Verification items for the finished model (mm, model axes). A direction names the side the tool comes from. Give positions to 0.01 mm unless a question says otherwise; leave off trailing zeros. Loops run counter-clockwise (first coordinate to the right, second up) from the corner with the lowest first, then second, coordinate; pieces in that order, holes last. Notation, with made-up numbers: M 82.25,-19.75 L 134.25,-19.75 A16 ccw 134.25,-1.75 Z; hole C 89,-36 d9. An arc over 180 degrees is marked long. Answer in a Markdown table with one row per item.
```python
from build123d import *

# Parameters (mm, degrees)
F0_R     = 17.5
F1_DEPTH = 2.5
F2_R     = 3
F3_DEPTH = 5


with BuildPart() as f1:
    # F0 (on Front) → F1 (new body, symmetric)
    with BuildSketch(Plane.XZ):
        Circle(F0_R)
        with BuildLine():
            ThreePointArc((-3.4692543384, -12.0089247785), (-6.25, -10.8253175473), (-8.6654067611, -9.0089247785))
            Line((-8.6654067611, -9.0089247785), (-7.8895788335, -7.6651513899))
            ThreePointArc((-7.8895788335, -7.6651513899), (-9.5262794416, -5.5), (-10.5830052443, -3))
            Line((-10.5830052443, -3), (-12.1346610995, -3))
            ThreePointArc((-12.1346610995, -3), (-12.5, 0), (-12.1346610995, 3))
            Line((-12.1346610995, 3), (-10.5830052443, 3))
            ThreePointArc((-10.5830052443, 3), (-9.5262794416, 5.5), (-7.8895788335, 7.6651513899))
            Line((-7.8895788335, 7.6651513899), (-8.6654067611, 9.0089247785))
            ThreePointArc((-8.6654067611, 9.0089247785), (-6.25, 10.8253175473), (-3.4692543384, 12.0089247785))
            Line((-3.4692543384, 12.0089247785), (-2.6934264108, 10.6651513899))
            ThreePointArc((-2.6934264108, 10.6651513899), (0, 11), (2.6934264108, 10.6651513899))
            Line((2.6934264108, 10.6651513899), (3.4692543384, 12.0089247785))
            ThreePointArc((3.4692543384, 12.0089247785), (6.25, 10.8253175473), (8.6654067611, 9.0089247785))
            Line((8.6654067611, 9.0089247785), (7.8895788335, 7.6651513899))
            ThreePointArc((7.8895788335, 7.6651513899), (9.5262794416, 5.5), (10.5830052443, 3))
            Line((10.5830052443, 3), (12.1346610995, 3))
            ThreePointArc((12.1346610995, 3), (12.5, 0), (12.1346610995, -3))
            Line((12.1346610995, -3), (10.5830052443, -3))
            ThreePointArc((10.5830052443, -3), (9.5262794416, -5.5), (7.8895788335, -7.6651513899))
            Line((7.8895788335, -7.6651513899), (8.6654067611, -9.0089247785))
            ThreePointArc((8.6654067611, -9.0089247785), (6.25, -10.8253175473), (3.4692543384, -12.0089247785))
            Line((3.4692543384, -12.0089247785), (2.6934264108, -10.6651513899))
            ThreePointArc((2.6934264108, -10.6651513899), (0, -11), (-2.6934264108, -10.6651513899))
            Line((-2.6934264108, -10.6651513899), (-3.4692543384, -12.0089247785))
        make_face(mode=Mode.SUBTRACT)
    extrude(amount=F1_DEPTH, both=True)

    # F2 (on face) → F3 (join, through all)
    with BuildSketch(Plane.XZ.offset(2.5)):
        with BuildLine():
            Line((-5.0203666831, 24.2857142857), (-14.642736159, 9.5833333333))
            ThreePointArc((-14.642736159, 9.5833333333), (0, 17.5), (14.642736159, 9.5833333333))
            Line((14.642736159, 9.5833333333), (5.0203666831, 24.2857142857))
            ThreePointArc((5.0203666831, 24.2857142857), (0, 27), (-5.0203666831, 24.2857142857))
        make_face()
        with Locations((0, 21)):
            Circle(F2_R, mode=Mode.SUBTRACT)
        with BuildLine():
            ThreePointArc((14.642736159, -9.5833333333), (0, -17.5), (-14.642736159, -9.5833333333))
            Line((-14.642736159, -9.5833333333), (-5.0203666831, -24.2857142857))
            ThreePointArc((-5.0203666831, -24.2857142857), (0, -27), (5.0203666831, -24.2857142857))
            Line((5.0203666831, -24.2857142857), (14.642736159, -9.5833333333))
        make_face()
        with Locations((0, -21)):
            Circle(F2_R, mode=Mode.SUBTRACT)
    extrude(amount=-F3_DEPTH)


solid = f1.part
```
Item 1: Sectioned sample at D-D (x = -7). Record the cut outline in (y, z).
Reported:
| item | result |
|---|---|
| outline | M -2.5,-21.26 L 2.5,-21.26 L 2.5,-10.36 L -2.5,-10.36 Z; M -2.5,10.36 L 2.5,10.36 L 2.5,21.26 L -2.5,21.26 Z |
Item 2: Tool access check on faces 5 (the flat face through (-9.9, -0.04, -16.83)), 6 (the cylindrical face through (12.5, 0, 0)). Record the directions out of +Z, -Z, +X, -X, +Y, -Y that give a thin tool (end or side, any length) a straight path to the whole face; none if there is none.
Reported:
| item | result |
|---|---|
| face 5 | -Z, -X, +Y, -Y |
| face 6 | +Y, -Y |
Item 3: Sectioned sample at C-C (z = 20). Record the cut outline in (x, y), and give its area (3 significant figures).
Reported:
| item | result |
|---|---|
| outline | M -7.83,-2.5 L -2.83,-2.5 L -2.83,2.5 L -7.83,2.5 Z; M 2.83,-2.5 L 7.83,-2.5 L 7.83,2.5 L 2.83,2.5 Z |
| area | 50.0 mm^2 |
Item 4: Scan lines: L1, parallel to Z at x = 0, y = -0.05; L2, parallel to Z at x = -1.5, y = -1.8; L3, parallel to X at y = -2.2, z = 7.5. Record each from-to range of solid material in increasing order. Write a range as [from, to].
Reported:
| item | result |
|---|---|
| L1 | z = [-27, -24], [-18, -11], [11, 18], [24, 27] |
| L2 | z = [-26.81, -23.6], [-18.4, -10.9], [10.9, 18.4], [23.6, 26.81] |
| L3 | x = [-15.81, -8.05], [8.05, 15.81] |
Item 5: Sectioned sample at B-B (x = 0). Record the cut outline in (y, z), and give its area (3 significant figures).
Reported:
| item | result |
|---|---|
| outline | M -2.5,-27 L 2.5,-27 L 2.5,-24 L -2.5,-24 Z; M -2.5,-18 L 2.5,-18 L 2.5,-11 L -2.5,-11 Z; M -2.5,11 L 2.5,11 L 2.5,18 L -2.5,18 Z; M -2.5,24 L 2.5,24 L 2.5,27 L -2.5,27 Z |
| area | 100 mm^2 |
Item 6: Sectioned sample at A-A (y = -1.6). State how many separate pieces and enclosed holes the cut face has, and give its area (3 significant figures).
Reported:
| item | result |
|---|---|
| separate pieces | 1 |
| enclosed holes | 3 |
| area | 761 mm^2 |
Item 7: Go/stop test with flat-tipped pins: pin 1 (1.2 mm diameter, centred on x = -11.5, y = 1, fed in from -Z); pin 2 (1 mm diameter, centred on x = 6.5, y = 1, fed in from +Z); pin 3 (1.2 mm diameter, centred on x = -11.5, y = 1, fed in from +Z). Record where each tip stops, or that it passes through.
Reported:
| item | result |
|---|---|
| pin 1 | stops at z = -15.3 |
| pin 2 | stops at z = 22.79 |
| pin 3 | stops at z = 15.3 |
Item 8: Release check for a two-part mould opening along Z. For faces 1 (the cylindrical face through (9.545, -0.035, -5.467)), 2 (the cylindrical face through (-6.21, -0.04, -10.85)), 3 (the flat face through (9.9, -0.04, 16.83)), 4 (the flat face through (0, 2.5, 12)) record: released by +Z, released by -Z, zero draft, split by the parting line, or undercut.
Reported:
| item | result |
|---|---|
| face 1 | undercut |
| face 2 | undercut |
| face 3 | released by +Z |
| face 4 | zero draft |
